Could you check a few things on this model? Use its own coordinates, in mm. A direction names the side the tool comes from. Give positions to 0.01 mm unless a question says otherwise; leave off trailing zeros. Loops run counter-clockwise (first coordinate to the right, second up) from the corner with the lowest first, then second, coordinate; pieces in that order, holes last.
1. Imagine slicing it at B-B (z = 10). List the corners of the cut face in (x, y) for me, plus the area to 3 significant figures.
2. For faces 1 (the flat face through (47, 1, 33)), 2 (the flat face through (47, 1, -29)), 3 (the flat face through (-1, 19, -38.5)), 4 (the flat face through (-53, 1, 0)), 5 (the flat face through (-43, 5, 32)), which set-ups out of +Z, -Z, +X, -X, +Y, -Y let a thin tool reach every point of the face, with its end or its side?
3. I need wall thicknesses on line 1 along Z through (x, y) = (-13, 3); line 2 along Z through (x, y) = (50.5, 14); line 3 along X through (y, z) = (18.5, -24). Which ranges of each line are inside material? Lowest first, please.
4. For P1, Ø4, axis at y = 5, z = -19.5, coming from the -X side; P2, Ø1.8, axis at x = -43.5, y = 13, coming from the -Z side; P3, Ø17.5, axis at x = 51, z = 5, coming from the +Y side, each with a flat end and sliding along its axis, tell me the tip position at first contact or that it passes through.
5. Imagine slicing it at A-A (y = 34). List the corners of the cut face in (x, z) for me.
6. Imagine slicing it at C-C (y = 22). List the corners of the cut face in (x, z) for me, plus the area to 3 significant figures.
7. Thinking about a two-plate mould opening in X: for faces 6 (the flat face through (47, 13, 28.5)), 7 (the cylindrical face through (46.41, 16.3, -38.01)), which applies, +X half, -X half, draft (parallel to the pull), parting line (faces both ways), or undercut?
```python
from build123d import *

# Parameters (mm, degrees)
ESBO_O1_W                = 111
ESBO_O1_H                = 77
RESSALTO_EXTRUS_O1_DEPTH = 1
ESBO_O2_W                = 111
ESBO_O2_H                = 1
RESSALTO_EXTRUS_O2_DEPTH = 36.7
ESBO_O3_W                = 90
ESBO_O3_H                = 76
RESSALTO_EXTRUS_O3_DEPTH = 36.7
ESBO_O4_W                = 16
ESBO_O4_H                = 49.2
RESSALTO_EXTRUS_O4_DEPTH = 24
ESBO_O5_R                = 1.15
CORTE_EXTRUS_O1_DEPTH    = 5
ESBO_O6_R                = 1.15
CORTE_EXTRUS_O2_DEPTH    = 5


with BuildPart() as part:
    # Esboço1 → Ressalto-extrusão1 (new body)
    with BuildSketch(Plane(origin=(0, 0, 0), x_dir=(1, 0, 0), z_dir=(0, 1, 0))):
        Rectangle(ESBO_O1_W, ESBO_O1_H)
    extrude(amount=RESSALTO_EXTRUS_O1_DEPTH)

    # Esboço2 → Ressalto-extrusão2 (add)
    with BuildSketch(Plane(origin=(0, 1, 0), x_dir=(1, 0, 0), z_dir=(0, 1, 0))):
        with Locations((0, 38)):
            Rectangle(ESBO_O2_W, ESBO_O2_H)
    extrude(amount=RESSALTO_EXTRUS_O2_DEPTH)

    # Esboço3 → Ressalto-extrusão3 (add)
    with BuildSketch(Plane(origin=(0, 1, 0), x_dir=(1, 0, 0), z_dir=(0, 1, 0))):
        with Locations((-5.5, -0.5)):
            Rectangle(ESBO_O3_W, ESBO_O3_H)
    extrude(amount=RESSALTO_EXTRUS_O3_DEPTH)

    # Esboço4 → Ressalto-extrusão4 (add)
    with BuildSketch(Plane(origin=(0, 1, 0), x_dir=(1, 0, 0), z_dir=(0, 1, 0))):
        with Locations((47.5, -3.9)):
            Rectangle(ESBO_O4_W, ESBO_O4_H)
    extrude(amount=RESSALTO_EXTRUS_O4_DEPTH)

    # Esboço5 → Corte-extrusão1 (cut)
    with BuildSketch(Plane(origin=(0, 0, -38.5), x_dir=(-1, 0, 0), z_dir=(0, 0, -1))):
        with Locations((-45.5, 17)):
            Circle(ESBO_O5_R)
        with Locations((43.5, 13)):
            Circle(ESBO_O5_R)
        with BuildLine():
            Line((55.5, 30.606515891), (52.6, 30.606515891))
            ThreePointArc((52.6, 30.606515891), (51, 29.006515891), (52.6, 27.406515891))
            Line((52.6, 27.406515891), (55.5, 27.406515891))
            Line((55.5, 27.406515891), (55.5, 30.606515891))
        make_face()
    extrude(amount=-CORTE_EXTRUS_O1_DEPTH, mode=Mode.SUBTRACT)

    # Esboço6 → Corte-extrusão2 (cut)
    with BuildSketch(Plane.XZ):
        with Locations((-42.5, 31.5)):
            Circle(ESBO_O6_R)
        with Locations((50.5, 33.5)):
            Circle(ESBO_O6_R)
        with Locations((-13, 13)):
            Circle(ESBO_O6_R)
        with Locations((23.5, 13.5)):
            Circle(ESBO_O6_R)
        with Locations((-13, -15)):
            Circle(ESBO_O6_R)
    extrude(amount=-CORTE_EXTRUS_O2_DEPTH, mode=Mode.SUBTRACT)


solid = part.part
```
Derived:
1. outline: (-55.5, 0) - (55.5, 0) - (55.5, 25) - (39.5, 25) - (39.5, 37.7) - (-50.5, 37.7) - (-50.5, 1) - (-55.5, 1) - close
1. area: 3,800 mm2
2. face 1: +Z, +X, +Y
2. face 2: +X, +Y
2. face 3: -Z, +X, -X, +Y, -Y
2. face 4: +Z, -X, +Y
2. face 5: -Y
3. line 1: z = -38.5 to -16.15, -13.85 to 11.85, 14.15 to 38.5
3. line 2: z = -38.5 to -37.5, -20.7 to 28.5
3. line 3: x = -50.5 to 39.5
4. P1: stops at x = -50.5
4. P2: stops at z = -33.5
4. P3: stops at y = 25
5. outline: (-55.5, -38.5) - (55.5, -38.5) - (55.5, -37.5) - (39.5, -37.5) - (39.5, 38.5) - (-50.5, 38.5) - (-50.5, -37.5) - (-55.5, -37.5) - close
6. outline: (-55.5, -38.5) - (55.5, -38.5) - (55.5, -37.5) - (39.5, -37.5) - (39.5, -20.7) - (55.5, -20.7) - (55.5, 28.5) - (39.5, 28.5) - (39.5, 38.5) - (-50.5, 38.5) - (-50.5, -37.5) - (-55.5, -37.5) - close
6. area: 7,740 mm2
7. face 6: draft
7. face 7: undercut
